from build123d import *

# Parameters (mm, degrees)
SKETCH1_W                   = 101.6
SKETCH1_H                   = 130.175
BOSS_EXTRUDE1_DEPTH         = 12.7
CUT_EXTRUDE1_DEPTH          = 87.383925914
CUT_EXTRUDE1_DEPTH_BACK     = 87.383925914
SKETCH2_R                   = 16.51
F_3_8_CLEARANCE_HOLE1_D     = 10.0838
F_1_4_20_TAPPED_HOLE1_D     = 5.1054
F_1_4_20_TAPPED_HOLE1_DEPTH = 16.51
F_1_4_20_TAPPED_HOLE1_TIP   = 1.533816902


with BuildPart() as part:
    # Sketch1 → Boss-Extrude1 (new, symmetric)
    with BuildSketch(Plane(origin=(0, 0, 0), x_dir=(1, 0, 0), z_dir=(0, 1, 0))):
        Rectangle(SKETCH1_W, SKETCH1_H)
    extrude(amount=BOSS_EXTRUDE1_DEPTH, both=True)

    # Sketch2 → Cut-Extrude1 (cut, two sides: drawn at the far end of the back side and taken through both)
    with BuildSketch(Plane(origin=(0, 12.7, 0), x_dir=(1, 0, 0), z_dir=(0, 1, 0)).offset(-CUT_EXTRUDE1_DEPTH_BACK)):
        with Locations(Location((-25.4, -14.2875, 0), (0, 0, 270))):
            Circle(SKETCH2_R)
    extrude(amount=CUT_EXTRUDE1_DEPTH + CUT_EXTRUDE1_DEPTH_BACK, mode=Mode.SUBTRACT)

    # 3/8 Clearance Hole1 (through all)
    with Locations(Plane(origin=(0, -12.7, 0), x_dir=(-1, 0, 0), z_dir=(0, -1, 0))):
        with Locations((-38.1, 50.8), (38.1, 50.8), (38.1, -50.8), (-38.1, -50.8)):
            Hole(F_3_8_CLEARANCE_HOLE1_D / 2)

    # 1/4-20 Tapped Hole1
    with Locations(Plane.ZY.offset(50.8)):
        with Locations((14.2875, 0)):
            Hole(F_1_4_20_TAPPED_HOLE1_D / 2, depth=F_1_4_20_TAPPED_HOLE1_DEPTH)
            with Locations((0, 0, -(F_1_4_20_TAPPED_HOLE1_DEPTH + F_1_4_20_TAPPED_HOLE1_TIP / 2))):  # 118° drill point
                Cone(0, F_1_4_20_TAPPED_HOLE1_D / 2, F_1_4_20_TAPPED_HOLE1_TIP, mode=Mode.SUBTRACT)


solid = part.part
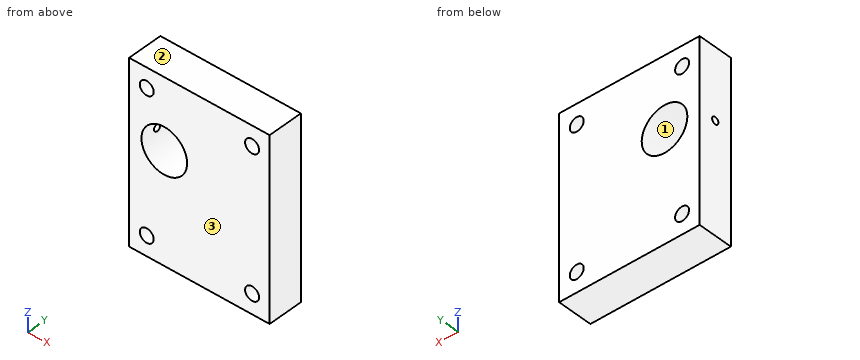
Design review of the part built by this model. Coordinates are the model's own, in mm. Face numbers are marked on the shaded views. Give positions to 0.01 mm unless a question says otherwise; leave off trailing zeros. Order: outer loops, then holes, each group sorted by start corner. A loop starts at its lowest first (then second) coordinate and runs counter-clockwise, first axis right, second up.
1. Add section A-A, the plane x = 38.1. State the section outline as (y, z) points, then the cut area to 3 significant figures.
Solution:
outline: (-12.7, -65.09) - (12.7, -65.09) - (12.7, -55.84) - (-12.7, -55.84) - close; (-12.7, -45.76) - (12.7, -45.76) - (12.7, 45.76) - (-12.7, 45.76) - close; (-12.7, 55.84) - (12.7, 55.84) - (12.7, 65.09) - (-12.7, 65.09) - close
area: 2,790 mm2
2. Add section B-B, the plane y = 10.5. State the section outline as (x, z) points.
Solution:
outline: (-50.8, -65.09) - (50.8, -65.09) - (50.8, 65.09) - (-50.8, 65.09) - close; hole circle Ø10.08 at (-38.1, -50.8); hole circle Ø10.08 at (-38.1, 50.8); hole circle Ø33.02 at (-25.4, 14.29); hole circle Ø10.08 at (38.1, -50.8); hole circle Ø10.08 at (38.1, 50.8)
3. Add section D-D, the plane x = -25.4. State the section outline as (y, z) points.
Solution:
outline: (-12.7, -65.09) - (12.7, -65.09) - (12.7, -2.22) - (-12.7, -2.22) - close; (-12.7, 30.8) - (12.7, 30.8) - (12.7, 65.09) - (-12.7, 65.09) - close
4. Mouldability with a two-part tool opening along Z and no side actions: class the marked faces 1, 2 and 3 as +Z half, -Z half, draft (parallel to the pull), parting line (faces both ways), or undercut.
Solution:
face 1: undercut
face 2: +Z half
face 3: draft
5. To check wall thickness, follow L1, parallel to Z at x = 38.1, y = -5; L2, parallel to X at y = -1, z = -50.8; L3, parallel to Z at x = -37, y = -8.25. State the ranges of each line that lie inside material, in increasing order.
Solution:
L1: z = -65.09 to -55.84, -45.76 to 45.76, 55.84 to 65.09
L2: x = -50.8 to -43.14, -33.06 to 33.06, 43.14 to 50.8
L3: z = -65.09 to -55.72, -45.88 to 2.54, 26.04 to 45.88, 55.72 to 65.09
6. For pin 1 Ø13 at (x, z) = (38.1, 50.8) entering from -Y; pin 2 Ø4 at (y, z) = (0, 14.29) entering from -X, all flat-tipped, find the tip position at first contact; note any pin that passes through.
Solution:
pin 1: stops at y = -12.7
pin 2: stops at x = -9.01
7. Add section C-C, the plane z = 50.8. State the section outline as (x, y) points.
Solution:
outline: (-50.8, -12.7) - (-43.14, -12.7) - (-43.14, 12.7) - (-50.8, 12.7) - close; (-33.06, -12.7) - (33.06, -12.7) - (33.06, 12.7) - (-33.06, 12.7) - close; (43.14, -12.7) - (50.8, -12.7) - (50.8, 12.7) - (43.14, 12.7) - close
